```python
from build123d import *

# Parameters (mm, degrees)
SKETCH1_R      = 3
EXTRUDE1_DEPTH = 4


with BuildPart() as part:
    # Sketch1 → Extrude1 (new body)
    with BuildSketch(Plane.XY):
        with BuildLine():
            Line((96.579798567, -9.396926208), (124.77057719, -19.657530508))
            Line((124.77057719, -19.657530508), (203.128908943, -76.403070631))
            ThreePointArc((203.128908943, -76.403070631), (206.658928298, -76.205679261), (206.461536928, -72.675659906))
            Line((206.461536928, -72.675659906), (131.610980057, -0.863678092))
            Line((131.610980057, -0.863678092), (103.420201433, 9.396926208))
            Line((103.420201433, 9.396926208), (-0.005150596, 5.749997693))
            ThreePointArc((-0.005150596, 5.749997693), (-5.74995391, -0.023022325), (0.040893831, -5.74985458))
            Line((0.040893831, -5.74985458), (96.579798567, -9.396926208))
        make_face()
        Circle(SKETCH1_R, mode=Mode.SUBTRACT)
        with Locations((100, 0)):
            Circle(SKETCH1_R, mode=Mode.SUBTRACT)
    extrude(amount=EXTRUDE1_DEPTH)


solid = part.part
```
For this review, take the finished solid that the model builds, in its own axes (mm). Coordinates: 2 decimals unless noted, no trailing zeros. Write each loop counter-clockwise with the first axis right and the second up, starting at its lowest first coordinate (ties: lowest second). Pieces come first, ordered by that corner, then holes. Notation, with made-up numbers: (75, 7.5) -> (107, 7.5) arc R6 cw to (107, 17.5) -> close; hole circle Ø7 at (30.5, -30.75). An arc over 180 degrees is marked (long way). Put each result on its own line as item: value.
Q1. The part is to be moulded in two halves that separate along X. For faces 1 (the cylindrical face through (206.62, -76.25, 1.97)), 2 (the cylindrical face through (-3, 0, 2)), 3 (the flat face through (110.478, -14.455, 1.972)), say which applies: +X half, -X half, draft (parallel to the pull), parting line (faces both ways), or undercut.
From the geometry:
face 1: parting line
face 2: undercut
face 3: -X half
Q2. Wall thickness on L1, parallel to Y at x = 0, z = 2.15; L2, parallel to Y at x = 100, z = 2.3; L3, parallel to X at y = -69.5, z = 0.45: over which ranges is each line inside the solid? List them lowest first.
From the geometry:
L1: y = -5.75 to -3, 3 to 5.75
L2: y = -10.64 to -3, 3 to 9.28
L3: x = 193.6 to 203.15
Q3. Take a section at C-C, the plane y = -25. State the section outline as (x, z) points, then the cut area to 3 significant figures.
From the geometry:
outline: (132.15, 0) -> (156.77, 0) -> (156.77, 4) -> (132.15, 4) -> close
area: 98.5 mm2
Q4. Take a section at A-A, the plane z = 0.9. State the section outline as (x, y) points.
From the geometry:
outline: (-0.01, 5.75) arc R5.75 ccw (long way) to (0.04, -5.75) -> (96.58, -9.4) -> (124.77, -19.66) -> (203.13, -76.4) arc R2.5 ccw to (206.46, -72.68) -> (131.61, -0.86) -> (103.42, 9.4) -> close; hole circle Ø6 at (0, 0); hole circle Ø6 at (100, 0)
Q5. Clearance check with flat-ended pins moving along their axes: pin 1 Ø1 at (x, z) = (131, 2) entering from -Y; pin 2 Ø2 at (y, z) = (-33.5, 2.5) entering from -X. State where each tip first meets the part, or that it passes through.
From the geometry:
pin 1: stops at y = -24.53
pin 2: stops at x = 142.5
Q6. Take a section at D-D, the plane x = 157.5. State the section outline as (y, z) points, then the cut area to 3 significant figures.
From the geometry:
outline: (-43.36, 0) -> (-25.7, 0) -> (-25.7, 4) -> (-43.36, 4) -> close
area: 70.6 mm2
Q7. Take a section at B-B, the plane x = 100. State the section outline as (y, z) points.
From the geometry:
outline: (-10.64, 0) -> (-3, 0) -> (-3, 4) -> (-10.64, 4) -> close; (3, 0) -> (9.28, 0) -> (9.28, 4) -> (3, 4) -> close
